Model file for the job. Use its own axes, mm. Round coordinates to 2 decimals unless told otherwise and drop trailing zeros. Order: outer loops, then holes, each group sorted by start corner. A loop starts at its lowest first (then second) coordinate and runs counter-clockwise, first axis right, second up. Notation, with made-up numbers: (47, -6) - (66, -6) arc R19 cw to (66, 6) - close; hole circle Ø4 at (70, -33.75). An arc over 180 degrees is marked (long way). Write item = value, one per line.
```python
from build123d import *

# Parameters (mm, degrees)
F0_W     = 914.4
F0_H     = 914.4
F0_W_2   = 876.3
F0_H_2   = 876.3
F1_DEPTH = 19.05
F3_DEPTH = 19.05


with BuildPart() as f1:
    # F0 (on Top) → F1 (new body)
    with BuildSketch(Plane.XY):
        Rectangle(F0_W, F0_H)
        Rectangle(F0_W_2, F0_H_2, mode=Mode.SUBTRACT)
    extrude(amount=F1_DEPTH)

    # F2 (on Top) → F3 (join)
    with BuildSketch(Plane.XY):
        Polygon((438.15, 257.175), (438.15, 276.225), (-438.15, 276.225), (-438.15, 257.175), (0, 257.175), align=None)
    extrude(amount=F3_DEPTH)


solid = f1.part
```
1) Cut at A-A (x = -31.5). Write the cut outline in (y, z) (3 decimals).
Conclusion:
outline = (-457.2, 0) - (-438.15, 0) - (-438.15, 19.05) - (-457.2, 19.05) - close; (257.175, 0) - (276.225, 0) - (276.225, 19.05) - (257.175, 19.05) - close; (438.15, 0) - (457.2, 0) - (457.2, 19.05) - (438.15, 19.05) - close
2) Wall check: line 1 along Y through (x, z) = (302.5, 1) (3 decimals); line 2 along X through (y, z) = (13.5, 14.75). Give the ranges that are in metal, low to high.
Conclusion:
line_1 = -457.2 to -438.15, 257.175 to 276.225, 438.15 to 457.2
line_2 = -457.2 to -438.15, 438.15 to 457.2
3) Cut at B-B (y = -2.5). Write the cut outline in (x, z), and give its area (3 significant figures).
Conclusion:
outline = (-457.2, 0) - (-438.15, 0) - (-438.15, 19.05) - (-457.2, 19.05) - close; (438.15, 0) - (457.2, 0) - (457.2, 19.05) - (438.15, 19.05) - close
area = 726 mm^2
4) Cut at C-C (z = 6.5). Write the cut outline in (x, y) (3 decimals), and give its area (3 significant figures).
Conclusion:
outline = (-457.2, -457.2) - (457.2, -457.2) - (457.2, 457.2) - (-457.2, 457.2) - close; hole (-438.15, -438.15) - (438.15, -438.15) - (438.15, 257.175) - (-438.15, 257.175) - close; hole (-438.15, 276.225) - (438.15, 276.225) - (438.15, 438.15) - (-438.15, 438.15) - close
area = 84,900 mm^2
